```python
from build123d import *

# Parameters (mm, degrees)
F0_W           = 135
F0_H           = 10
F1_DEPTH       = 25
F4_DEPTH       = 75
F6_DEPTH       = 3
F7_W           = 60
F7_H           = 15
F8_DEPTH       = 25
F9_D           = 13.2
F9_CBORE_D     = 23
F9_CBORE_DEPTH = 0


with BuildPart() as f1:
    # F0 (on Front) → F1 (new body, symmetric)
    with BuildSketch(Plane.XZ):
        Rectangle(F0_W, F0_H)
    extrude(amount=F1_DEPTH, both=True)

    # F3 (on face) → F4 (join)
    with BuildSketch(Plane.XY.offset(5)):
        Polygon((-60, 3.5), (-67.5, 3.5), (-67.5, -1.5), (-60, -1.5), (-60, -10), (-54.5, -10), (-54.5, 12), (-60, 12), align=None)
    extrude(amount=-F4_DEPTH)

    # F5 (on face) → F6 (join)
    with BuildSketch(Plane.XY.offset(5)):
        with BuildLine():
            ThreePointArc((-28.172621, 0), (-23.265569, 5.693772), (-21.5, 13))
            ThreePointArc((-21.5, 13), (-44.806228, 27.234431), (-46.827379, 0))
            ThreePointArc((-46.827379, 0), (-37.5, 3), (-28.172621, 0))
        make_face()
        with BuildLine():
            ThreePointArc((-28.172621, 0), (-37.5, -3), (-46.827379, 0))
            ThreePointArc((-46.827379, 0), (-44.806228, -27.234431), (-21.5, -13))
            ThreePointArc((-21.5, -13), (-23.265569, -5.693772), (-28.172621, 0))
        make_face()
    extrude(amount=-F6_DEPTH)

    # F7 (on face) → F8 (cut)
    with BuildSketch(Plane(origin=(0, 0, -5), x_dir=(1, 0, 0), z_dir=(0, 0, -1))):
        with Locations((12.5, 17.5)):
            Rectangle(F7_W, F7_H)
        with Locations((12.5, -17.5)):
            Rectangle(F7_W, F7_H)
    extrude(amount=-F8_DEPTH, mode=Mode.SUBTRACT)

    # F9 (through all)
    with Locations(Plane(origin=(0, 0, -5), x_dir=(1, 0, 0), z_dir=(0, 0, -1))):
        with Locations((-37.5, 13), (-37.5, -13)):
            CounterBoreHole(F9_D / 2, F9_CBORE_D / 2, F9_CBORE_DEPTH)


solid = f1.part
```
Build history of the part. All positions in model axes, mm. A direction names the side the tool comes from. Give positions to 0.01 mm unless a question says otherwise; leave off trailing zeros. Loops run counter-clockwise (first coordinate to the right, second up) from the corner with the lowest first, then second, coordinate; pieces in that order, holes last. Notation, with made-up numbers: (11.5, 59.25) - (40.5, 59.25) arc R30 cw to (40.5, 81.25) - close; hole circle Ø5 at (-10.5, 83). An arc over 180 degrees is marked (long way). Use a Markdown table: item, result.
(1) Band-saw the part on C-C (x = -37.5). Give the cut face in (y, z).
Taken from the geometry:
| item | result |
|---|---|
| outline | (-29, 2) - (-25, 2) - (-25, -5) - (-19.6, -5) - (-19.6, 5) - (-29, 5) - close; (-6.4, -5) - (6.4, -5) - (6.4, 5) - (-6.4, 5) - close; (19.6, -5) - (25, -5) - (25, 2) - (29, 2) - (29, 5) - (19.6, 5) - close |
(2) Wall check: line 1 along Y through (x, z) = (-37.5, -0.5); line 2 along Z through (x, y) = (52.5, 19.5); line 3 along X through (y, z) = (11, -43). Give the ranges that are in metal, low to high.
Taken from the geometry:
| item | result |
|---|---|
| line 1 | -25 to -19.6, -6.4 to 6.4, 19.6 to 25 |
| line 2 | -5 to 5 |
| line 3 | -60 to -54.5 |
(3) Band-saw the part on A-A (y = -13). Give the cut face in (x, z), and give its area (3 significant figures).
Taken from the geometry:
| item | result |
|---|---|
| outline | (-67.5, -5) - (-44.1, -5) - (-44.1, 5) - (-67.5, 5) - close; (-30.9, -5) - (-17.5, -5) - (-17.5, 5) - (-30.9, 5) - close; (42.5, -5) - (67.5, -5) - (67.5, 5) - (42.5, 5) - close |
| area | 618 mm2 |
(4) Pull direction X, two halves, no side cores. Call faces 1 (the face through (-67.5, 0, -13)), 2 (the face through (55, -25, 0)), 3 (the face through (-43.597, 15.528, 0.07)): +X half, -X half, draft (parallel to the pull), parting line (faces both ways), or undercut.
Taken from the geometry:
| item | result |
|---|---|
| face 1 | -X half |
| face 2 | draft |
| face 3 | undercut |
(5) Band-saw the part on D-D (z = -48). Give the cut face in (x, y), and give its area (4 significant figures).
Taken from the geometry:
| item | result |
|---|---|
| outline | (-67.5, -1.5) - (-60, -1.5) - (-60, -10) - (-54.5, -10) - (-54.5, 12) - (-60, 12) - (-60, 3.5) - (-67.5, 3.5) - close |
| area | 158.5 mm2 |
(6) Which spindle directions (+Z, -Z, +X, -X, +Y, -Y) get a long thin tool onto all of the face, cutting with end or side? Do faces 4 (the face through (-60, -6, -37)), 5 (the face through (-17.5, 18, 0)), 6 (the face through (55, 25, 0)). Say none if no direction does.
Taken from the geometry:
| item | result |
|---|---|
| face 4 | -Z, -X, -Y |
| face 5 | +Z, -Z, +Y |
| face 6 | +Z, -Z, +X, +Y |
(7) Band-saw the part on B-B (y = 22). Give the cut face in (x, z).
Taken from the geometry:
| item | result |
|---|---|
| outline | (-67.5, -5) - (-17.5, -5) - (-17.5, 5) - (-67.5, 5) - close; (42.5, -5) - (67.5, -5) - (67.5, 5) - (42.5, 5) - close |
(8) Drop flat-ended pins along their axis: pin 1 Ø8 at (x, z) = (-64.5, -28.5) entering from -Y; pin 2 Ø6.5 at (y, z) = (3.5, -47) entering from +X; pin 3 Ø6 at (y, z) = (12, -35) entering from -X. Give the stop position or say it passes through.
Taken from the geometry:
| item | result |
|---|---|
| pin 1 | y = -1.5 |
| pin 2 | x = -54.5 |
| pin 3 | x = -60 |
